Model file for the job. Use its own axes, mm. Round coordinates to 2 decimals unless told otherwise and drop trailing zeros. Loops run counter-clockwise (first coordinate to the right, second up) from the corner with the lowest first, then second, coordinate; pieces in that order, holes last. Notation, with made-up numbers: (55.5, -1.75) -> (72.5, -1.75) arc R11 cw to (72.5, 3.25) -> close; hole circle Ø11 at (41, 6.5). An arc over 180 degrees is marked (long way). Use a Markdown table: item, result.
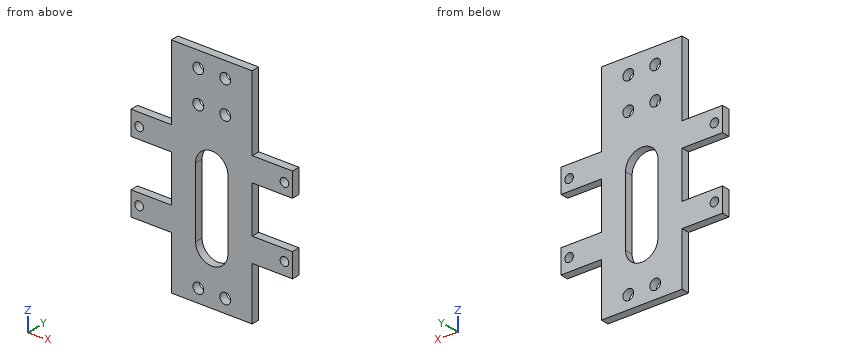
from build123d import *

# Parameters (mm, degrees)
EXTRUDE_1_DEPTH     = 3
SKETCH_2_R          = 1.6
CUT_EXTRUDE_1_DEPTH = 3
SKETCH_3_R          = 2
CUT_EXTRUDE_2_DEPTH = 3
CUT_EXTRUDE_3_DEPTH = 3


with BuildPart() as part:
    # 草图1 → 凸台-拉伸1 (new body)
    with BuildSketch(Plane(origin=(0, 0, 0), x_dir=(1, 0, 0), z_dir=(0, 1, 0))):
        Polygon((0, 0), (15, 0), (15, -28), (45, -28), (45, 0), (60, 0), (60, 9), (45, 9), (45, 26.6), (60, 26.6), (60, 35.6), (45, 35.6), (45, 55.6), (15, 55.6), (15, 35.6), (0, 35.6), (0, 26.6), (15, 26.6), (15, 9), (0, 9), align=None)
    extrude(amount=EXTRUDE_1_DEPTH)

    # 草图2 → 切除-拉伸1 (cut)
    with BuildSketch(Plane(origin=(0, 3, 0), x_dir=(1, 0, 0), z_dir=(0, 1, 0))):
        with Locations(Location((3, 4.75, 0), (0, 0, 270))):
            Circle(SKETCH_2_R)
        with Locations(Location((3, 30.85, 0), (0, 0, 270))):
            Circle(SKETCH_2_R)
        with Locations(Location((57, 30.85, 0), (0, 0, 270))):
            Circle(SKETCH_2_R)
        with Locations(Location((57, 4.75, 0), (0, 0, 270))):
            Circle(SKETCH_2_R)
    extrude(amount=-CUT_EXTRUDE_1_DEPTH, mode=Mode.SUBTRACT)

    # 草图3 → 切除-拉伸2 (cut)
    with BuildSketch(Plane(origin=(0, 3, 0), x_dir=(1, 0, 0), z_dir=(0, 1, 0))):
        with Locations(Location((25, 50.6, 0), (0, 0, 270))):
            Circle(SKETCH_3_R)
        with Locations(Location((35, 50.6, 0), (0, 0, 270))):
            Circle(SKETCH_3_R)
        with Locations(Location((35, -22, 0), (0, 0, 270))):
            Circle(SKETCH_3_R)
        with Locations(Location((25, -22, 0), (0, 0, 270))):
            Circle(SKETCH_3_R)
        with Locations(Location((25, -10, 0), (0, 0, 270))):
            Circle(SKETCH_3_R)
        with Locations(Location((35, -10, 0), (0, 0, 270))):
            Circle(SKETCH_3_R)
    extrude(amount=-CUT_EXTRUDE_2_DEPTH, mode=Mode.SUBTRACT)

    # 草图4 → 切除-拉伸3 (cut)
    with BuildSketch(Plane(origin=(0, 3, 0), x_dir=(1, 0, 0), z_dir=(0, 1, 0))):
        with BuildLine():
            Line((36, 35.6), (36, 9.6))
            ThreePointArc((36, 9.6), (30, 3.6), (24, 9.6))
            Line((24, 9.6), (24, 35.6))
            ThreePointArc((24, 35.6), (30, 41.6), (36, 35.6))
        make_face()
    extrude(amount=-CUT_EXTRUDE_3_DEPTH, mode=Mode.SUBTRACT)


solid = part.part
Q1. Drill centre lines: L1, parallel to X at y = 1.4, z = -30.85; L2, parallel to X at y = 1.2, z = 22; L3, parallel to Z at x = 45.5, y = 1.35. Where is each one in solid material? Low to high. Write a range as from..to.
Results list:
| item | result |
|---|---|
| L1 | x = 0..1.4, 4.6..24, 36..55.4, 58.6..60 |
| L2 | x = 15..23, 27..33, 37..45 |
| L3 | z = -35.6..-26.6, -9..0 |
Q2. Band-saw the part on B-B, the plane y = 1. Give the number of separate pieces and of enclosed holes in the cut face, plus the area to 3 significant figures.
Results list:
| item | result |
|---|---|
| separate pieces | 1 |
| enclosed holes | 11 |
| area | 2,520 mm² |
Q3. Band-saw the part on D-D, the plane x = 30. Give the cut face in (y, z), plus the area to 3 significant figures.
Results list:
| item | result |
|---|---|
| outline | (0, -55.6) -> (3, -55.6) -> (3, -41.6) -> (0, -41.6) -> close; (0, -3.6) -> (3, -3.6) -> (3, 28) -> (0, 28) -> close |
| area | 137 mm² |
Q4. Band-saw the part on A-A, the plane z = 10. Give the cut face in (x, y).
Results list:
| item | result |
|---|---|
| outline | (15, 0) -> (23, 0) -> (23, 3) -> (15, 3) -> close; (27, 0) -> (33, 0) -> (33, 3) -> (27, 3) -> close; (37, 0) -> (45, 0) -> (45, 3) -> (37, 3) -> close |
Q5. Band-saw the part on C-C, the plane x = 3. Give the cut face in (y, z).
Results list:
| item | result |
|---|---|
| outline | (0, -35.6) -> (3, -35.6) -> (3, -32.45) -> (0, -32.45) -> close; (0, -29.25) -> (3, -29.25) -> (3, -26.6) -> (0, -26.6) -> close; (0, -9) -> (3, -9) -> (3, -6.35) -> (0, -6.35) -> close; (0, -3.15) -> (3, -3.15) -> (3, 0) -> (0, 0) -> close |
Q6. Flat gauge pins, fed straight in: pin 1 (3 mm diameter, centred on x = 25, z = -50.6, fed in from -Y); pin 2 (0.9 mm diameter, centred on x = 4, y = 1.5, fed in from -Z); pin 3 (1.5 mm diameter, centred on x = 55, y = 1.5, fed in from +Z); pin 4 (0.9 mm diameter, centred on y = 1.5, z = -15, fed in from -X). Where does each tip first touch, or does it go through?
Results list:
| item | result |
|---|---|
| pin 1 | passes through |
| pin 2 | stops at z = -35.6 |
| pin 3 | stops at z = 0 |
| pin 4 | stops at x = 15 |
